Design review of the part built by this model. Coordinates are the model's own, in mm. A direction names the side the tool comes from. Give positions to 0.01 mm unless a question says otherwise; leave off trailing zeros. Loops run counter-clockwise (first coordinate to the right, second up) from the corner with the lowest first, then second, coordinate; pieces in that order, holes last. Notation, with made-up numbers: M 64,-33 L 85,-33 A36 cw 85,1 Z; hole C 45.5,17.5 d8. An arc over 180 degrees is marked long. Answer as CSV lines item,"result".
```python
from build123d import *

# Parameters (mm, degrees)
F0_R          = 76.2
F1_DEPTH      = 158.28
F2_T          = -0.8
F3_R          = 1
F4_DEPTH      = 0.8
F5_W          = 8
F5_H          = 2
F6_DEPTH      = 76.201
F6_DEPTH_BACK = 76.201
F7_W          = 8
F7_H          = 4
F8_DEPTH      = 76.201
F8_DEPTH_BACK = 76.201


with BuildPart() as f1:
    # F0 (on Top) → F1 (new body)
    with BuildSketch(Plane.XY):
        Circle(F0_R)
    extrude(amount=F1_DEPTH)

    # F2
    f2_openings = [f1.faces().sort_by_distance(p)[0] for p in [
        (0, 0, 158.28),
    ]]
    offset(amount=F2_T, openings=f2_openings)

    # F3 (on face) → F4 (cut, through all)
    with BuildSketch(Plane.XY.offset(0.8)):
        Circle(F3_R)
    extrude(amount=-F4_DEPTH, mode=Mode.SUBTRACT)

    # F5 (on Front) → F6 (cut, two sides)
    with BuildSketch(Plane.XZ) as f6_sk:
        with Locations((0, 157.28)):
            Rectangle(F5_W, F5_H)
    extrude(amount=-F6_DEPTH, mode=Mode.SUBTRACT)
    extrude(f6_sk.sketch, amount=F6_DEPTH_BACK, mode=Mode.SUBTRACT)

    # F7 (on Right) → F8 (cut, two sides)
    with BuildSketch(Plane.YZ) as f8_sk:
        with Locations((0, 156.28)):
            Rectangle(F7_W, F7_H)
    extrude(amount=-F8_DEPTH, mode=Mode.SUBTRACT)
    extrude(f8_sk.sketch, amount=F8_DEPTH_BACK, mode=Mode.SUBTRACT)

    # F9 (on Front) → F10 (revolve)
    with BuildSketch(Plane.XZ):
        Polygon((76.2, 0.8), (76.2, 0), (100.8, 0), (100.8, -9.2), (101.6, -9.2), (101.6, 0.8), align=None)
    revolve(axis=Axis((0, 0, 18.5718685389), (0, 0, 1)))


solid = f1.part
```
1. For P1, Ø0.5, axis at x = -1.5, y = 75.5, coming from the +Z side; P2, Ø6, axis at y = 25, z = 20, coming from the -X side; P3, Ø1.5, axis at x = 78, y = 1, coming from the -Z side, all flat-tipped, find the tip position at first contact; note any pin that passes through.
Answer block:
P1,"z = 156.28"
P2,"x = -72.96"
P3,"z = 0"
2. To check wall thickness, follow L1, parallel to Y at x = 0, z = 99; L2, parallel to Y at x = 0, z = -5. State the ranges of each line that lie inside material, in increasing order. Write a range as [from, to].
Answer block:
L1,"[-76.2, -75.4], [75.4, 76.2]"
L2,"[-101.6, -100.8], [100.8, 101.6]"
3. We need section B-B, the plane z = 29. Write out the cut boundary in (x, y).
Answer block:
outline,"C 0,0 d152.4; hole C 0,0 d150.8"
4. For faces 1 (the flat face through (-1, 1, 0.8)), 2 (the cylindrical face through (-79.99, -61.34, -4.66)), 3 (the flat face through (-53.6, 53.6, 158.28)), list the 3-axis set-ups (+Z, -Z, +X, -X, +Y, -Y) from which the entire face can be reached by the end or side of a thin tool; tool diameter is ignored.
Answer block:
face 1,"+Z"
face 2,"-Z"
face 3,"+Z, +X, -X, +Y, -Y"
5. We need section D-D, the plane y = -84.5. Write out the cut boundary in (x, z).
Answer block:
outline,"M -56.41,-9.2 L -54.96,-9.2 L -54.96,0 L 54.96,0 L 54.96,-9.2 L 56.41,-9.2 L 56.41,0.8 L -56.41,0.8 Z"
6. The part is to be moulded in two halves that separate along Y. For faces 4 (the cylindrical face through (-22.025, -99.184, -4.13)), 5 (the flat face through (1, 1, 0)), 6 (the flat face through (-58.9, -47.9, 158.28)), say which applies: pulls with the +Y half, pulls with the -Y half, needs draft (parallel to the pull), parting line crosses it, or undercut.
Answer block:
face 4,"parting line crosses it"
face 5,"undercut"
face 6,"needs draft"
7. We need section C-C, the plane y = 25. Write out the cut boundary in (x, z), plus the area to 3 significant figures.
Answer block:
outline,"M -98.48,-9.2 L -97.65,-9.2 L -97.65,0 L 97.65,0 L 97.65,-9.2 L 98.48,-9.2 L 98.48,0.8 L 71.98,0.8 L 71.98,158.28 L 71.13,158.28 L 71.13,0.8 L -71.13,0.8 L -71.13,158.28 L -71.98,158.28 L -71.98,0.8 L -98.48,0.8 Z"
area,"440 mm²"
8. We need section A-A, the plane x = 53.5. Write out the cut boundary in (y, z).
Answer block:
outline,"M -86.37,-9.2 L -85.43,-9.2 L -85.43,0 L 85.43,0 L 85.43,-9.2 L 86.37,-9.2 L 86.37,0.8 L 54.26,0.8 L 54.26,158.28 L 53.13,158.28 L 53.13,0.8 L -53.13,0.8 L -53.13,158.28 L -54.26,158.28 L -54.26,0.8 L -86.37,0.8 Z"
